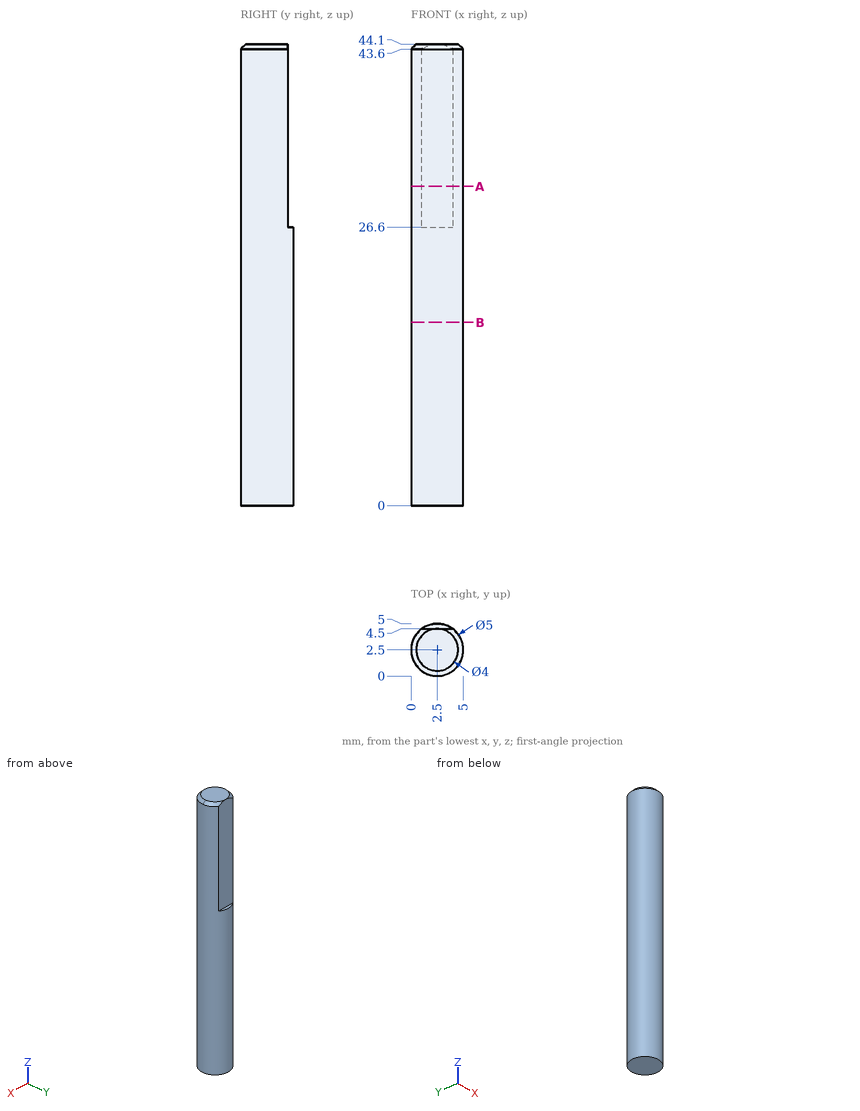
The drawing under review shows one solid part. Ordinate dimensions are in mm from its lowest x, y, z. Coordinates: 2 decimals unless noted, no trailing zeros. Write each loop counter-clockwise with the first axis right and the second up, starting at its lowest first coordinate (ties: lowest second). Pieces come first, ordered by that corner, then holes. Notation, with made-up numbers: (82.25, -7.75) - (108.25, -7.75) arc R14 cw to (108.25, 9.25) - close; hole circle Ø5 at (18.25, -27). An arc over 180 degrees is marked (long way). Answer as CSV lines item,"result".
(1) We need section B-B (z = 17.5). Give the boundary of the cut face in (x, y), plus the area to 3 significant figures.
Data:
outline,"circle Ø5 at (2.5, 2.5)"
area,"19.6 mm2"
(2) For line 1 along Y through (x, z) = (0.5, 37.5); line 2 along X through (y, z) = (4.65, 9); line 3 along Y through (x, z) = (2.35, 23.5), list the stretches that pass through material, from the lowest coordinate up. Write a range as [from, to].
Data:
line 1,"y = [1, 4]"
line 2,"x = [1.22, 3.78]"
line 3,"y = [0, 5]"
(3) We need section A-A (z = 30.5). Give the boundary of the cut face in (x, y).
Data:
outline,"(1, 4.5) arc R2.5 ccw (long way) to (4, 4.5) - close"
(4) Clearance check with flat-ended pins moving along their axes: pin 1 Ø1 at (y, z) = (4.5, 34.5) entering from -X; pin 2 Ø1 at (x, z) = (0.5, 33) entering from -Y; pin 3 Ø2 at (x, z) = (4.5, 20.5) entering from +Y. State where each tip first meets the part, or that it passes through.
Data:
pin 1,"stops at x = 0.5"
pin 2,"stops at y = 0.5"
pin 3,"stops at y = 4.79"
